CAD build for the part. Positions are in the model's coordinates, mm. A direction names the side the tool comes from. Coordinates: 2 decimals unless noted, no trailing zeros. Loops run counter-clockwise (first coordinate to the right, second up) from the corner with the lowest first, then second, coordinate; pieces in that order, holes last.
1) Two-plate mould, pull along Y, no slides. Class faces 1 (the flat face through (-16, -1, 2)), 2 (the flat face through (-17, 10, 0)), 3 (the flat face through (-19, 17.5, 6)): +Y half, -Y half, draft (parallel to the pull), parting line (faces both ways), or undercut.
2) Saw through at C-C, the plane z = 8.25. Write the cut outline in (x, y), and give its area (3 significant figures).
3) Which spindle directions (+Z, -Z, +X, -X, +Y, -Y) get a long thin tool onto all of the face, cutting with end or side? Do faces 4 (the flat face through (13, -1, 2.25)), 5 (the flat face through (6, -11, -2)), 6 (the flat face through (0, 0, 3.75)), 7 (the flat face through (-13, 11.5, 3)). Say none if no direction does.
4) Saw through at A-A, the plane z = 10.75. Write the cut outline in (x, y), and give its area (3 significant figures).
5) Saw through at B-B, the plane x = -19. Write the cut outline in (y, z), and give its area (3 significant figures).
6) Saw through at D-D, the plane x = -12. Write the cut outline in (y, z).
7) Wall check: line 1 along X through (y, z) = (16.6, 8.25); line 2 along X through (y, z) = (15, 0.5); line 3 along Y through (x, z) = (-14.5, 2.75). Give the ranges that are in metal, low to high.
8) Pin check, flat tips, straight feed: pin 1 Ø3.5 at (x, y) = (19.5, -3) entering from -Z; pin 2 Ø3 at (x, z) = (-1, 3) entering from +Y; pin 3 Ø2.5 at (x, y) = (-13, -2.5) entering from -Z. Stop position of each tip, or through.
```python
from build123d import *

# Parameters (mm, degrees)
BOSS_EXTRUDE1_DEPTH = 2.25
SKETCH2_W           = 12
SKETCH2_H           = 10
SKETCH2_R           = 1.5
BOSS_EXTRUDE3_DEPTH = 3
SKETCH3_W           = 5
SKETCH3_H           = 1
CUT_EXTRUDE1_DEPTH  = 19
SKETCH4_W           = 50
SKETCH4_H           = 23
BOSS_EXTRUDE5_DEPTH = 1.5
SKETCH5_W           = 10
SKETCH5_H           = 3.75
CUT_EXTRUDE2_DEPTH  = 4
SKETCH7_W           = 12
SKETCH7_H           = 2
BOSS_EXTRUDE6_DEPTH = 5
BOSS_EXTRUDE7_START = -1
SKETCH8_W           = 17
SKETCH8_H           = 2
BOSS_EXTRUDE7_DEPTH = 2.25


with BuildPart() as part:
    # Sketch1 → Boss-Extrude1 (new body)
    with BuildSketch(Plane.XY):
        Polygon((25, -11.5), (-25, -11.5), (-25, 11.5), (-25, 17.5), (-10.25, 17.5), (-10.25, 11.5), (10.25, 11.5), (10.25, 17.5), (25, 17.5), (25, 11.5), align=None)
    extrude(amount=BOSS_EXTRUDE1_DEPTH)

    # Sketch2 → Boss-Extrude3 (add)
    # profile 1 of 2: a face of its own
    with BuildSketch(Plane(origin=(0, 17.5, 0), x_dir=(1, 0, 0), z_dir=(0, 1, 0))):
        with Locations((19, -7.25)):
            Rectangle(SKETCH2_W, SKETCH2_H)
        with Locations(Location((19, -8.25, 0), (0, 0, 270))):
            Circle(SKETCH2_R, mode=Mode.SUBTRACT)
    # profile 2 of 2: a face of its own
    with BuildSketch(Plane(origin=(0, 17.5, 0), x_dir=(1, 0, 0), z_dir=(0, 1, 0))):
        with Locations((-19, -7.25)):
            Rectangle(SKETCH2_W, SKETCH2_H)
        with Locations(Location((-19, -8.25, 0), (0, 0, 90))):
            Circle(SKETCH2_R, mode=Mode.SUBTRACT)
    extrude(amount=-BOSS_EXTRUDE3_DEPTH)

    # Sketch3 → Cut-Extrude1 (cut)
    with BuildSketch(Plane.XZ.offset(11.5)):
        Polygon((-23, 1.25), (-23, 0), (23, 0), (23, 1.25), (16, 1.25), (11, 1.25), (-11, 1.25), (-16, 1.25), align=None)
        with Locations((-13.5, 1.75)):
            Rectangle(SKETCH3_W, SKETCH3_H)
        with Locations((13.5, 1.75)):
            Rectangle(SKETCH3_W, SKETCH3_H)
    extrude(amount=-CUT_EXTRUDE1_DEPTH, mode=Mode.SUBTRACT)

    # Sketch4 → Boss-Extrude5 (add)
    with BuildSketch(Plane.XY.offset(2.25)):
        Rectangle(SKETCH4_W, SKETCH4_H)
    extrude(amount=BOSS_EXTRUDE5_DEPTH)

    # Sketch5 → Cut-Extrude2 (cut)
    with BuildSketch(Plane(origin=(0, 11.5, 0), x_dir=(1, 0, 0), z_dir=(0, 1, 0))):
        with Locations((0, -1.875)):
            Rectangle(SKETCH5_W, SKETCH5_H)
    extrude(amount=-CUT_EXTRUDE2_DEPTH, mode=Mode.SUBTRACT)

    # Sketch7 → Boss-Extrude6 (add)
    with BuildSketch(Plane(origin=(0, 0, 1.25), x_dir=(-1, 0, 0), z_dir=(0, 0, -1))):
        with Locations((0, -10.5)):
            Rectangle(SKETCH7_W, SKETCH7_H)
    extrude(amount=BOSS_EXTRUDE6_DEPTH)

    # Sketch8 → Boss-Extrude7 (add)
    with BuildSketch(Plane(origin=(0, 0, 1.25), x_dir=(-1, 0, 0), z_dir=(0, 0, -1)).offset(BOSS_EXTRUDE7_START)):
        with Locations((14.5, -10.5)):
            Rectangle(SKETCH8_W, SKETCH8_H)
        with Locations((-14.5, -10.5)):
            Rectangle(SKETCH8_W, SKETCH8_H)
    extrude(amount=BOSS_EXTRUDE7_DEPTH)


solid = part.part
```
Data:
1. face 1: undercut
1. face 2: draft
1. face 3: +Y half
2. outline: (-25, 14.5) - (-20.5, 14.5) - (-20.5, 17.5) - (-25, 17.5) - close; (-17.5, 14.5) - (-13, 14.5) - (-13, 17.5) - (-17.5, 17.5) - close; (13, 14.5) - (17.5, 14.5) - (17.5, 17.5) - (13, 17.5) - close; (20.5, 14.5) - (25, 14.5) - (25, 17.5) - (20.5, 17.5) - close
2. area: 54.0 mm2
3. face 4: -Z
3. face 5: -Z, +X, +Y, -Y
3. face 6: +Z, +X, -X, -Y
3. face 7: +Z
4. outline: (-25, 14.5) - (-13, 14.5) - (-13, 17.5) - (-25, 17.5) - close; (13, 14.5) - (25, 14.5) - (25, 17.5) - (13, 17.5) - close
4. area: 72.0 mm2
5. outline: (-11.5, 0) - (-9.5, 0) - (-9.5, 1.25) - (7.5, 1.25) - (7.5, 0) - (17.5, 0) - (17.5, 6.75) - (14.5, 6.75) - (14.5, 2.25) - (11.5, 2.25) - (11.5, 3.75) - (-11.5, 3.75) - close; (14.5, 9.75) - (17.5, 9.75) - (17.5, 12.25) - (14.5, 12.25) - close
5. area: 99.5 mm2
6. outline: (-11.5, 0) - (-9.5, 0) - (-9.5, 2.25) - (7.5, 2.25) - (7.5, 0) - (17.5, 0) - (17.5, 2.25) - (11.5, 2.25) - (11.5, 3.75) - (-11.5, 3.75) - close
7. line 1: x = -25 to -20.5, -17.5 to -13, 13 to 17.5, 20.5 to 25
7. line 2: x = -25 to -10.25, 10.25 to 25
7. line 3: y = -11.5 to 11.5, 14.5 to 17.5
8. pin 1: stops at z = 1.25
8. pin 2: stops at y = 7.5
8. pin 3: stops at z = 2.25
